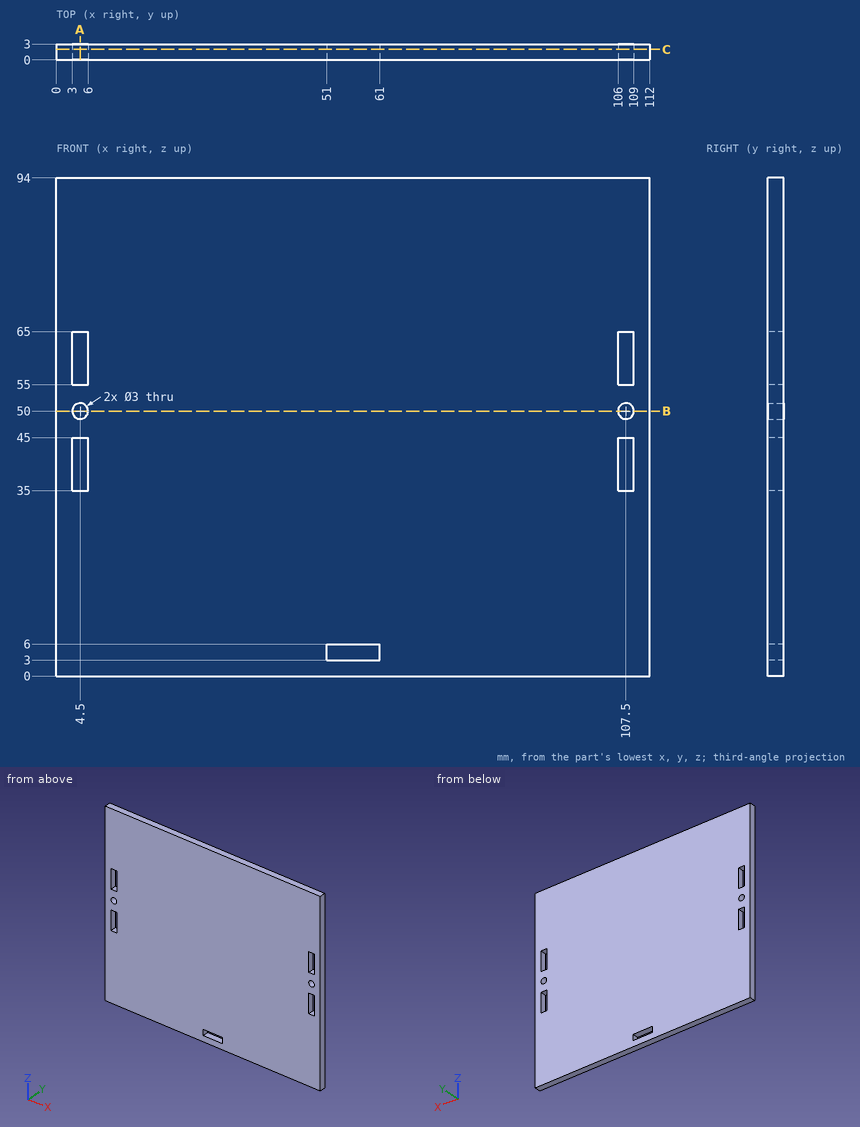
Geometry check sheet. Reference: drawing and pictorial views, mm from the part's lowest x, y, z. Round coordinates to 2 decimals unless told otherwise and drop trailing zeros. Loops run counter-clockwise (first coordinate to the right, second up) from the corner with the lowest first, then second, coordinate; pieces in that order, holes last. Notation, with made-up numbers: (-10.5, 12.25) -> (23.5, 12.25) arc R18 cw to (23.5, 25.25) -> close; hole circle Ø11 at (25, 54.5). An arc over 180 degrees is marked (long way). Answer as a JSON object with one key per item and string values. Group by question number.
Item 1: Depth check by flat-ended pin: pin 1 Ø1.8 at (x, z) = (107.5, 50) entering from +Y. Enter the tip coordinate at first touch or a pass-through.
Item 2: Cross-section at B-B, the plane z = 50. Record the cut outline in (x, y).
Item 3: Cross-section at C-C, the plane y = 2. Record the cut outline in (x, z).
Item 4: Cross-section at A-A, the plane x = 4.5. Record the cut outline in (y, z), plus the area to 3 significant figures.
Item 5: Thickness scan on line 1 along X through (y, z) = (2.2, 60.5); line 2 along Z through (x, y) = (4.5, 2.3); line 3 along Z through (x, y) = (55.5, 2.35). Record the ranges inside material, lowest first.
Determined:
{
 "1": {"pin 1": "passes through"},
 "2": {"outline": "(0, 0) -> (3, 0) -> (3, 3) -> (0, 3) -> close; (6, 0) -> (106, 0) -> (106, 3) -> (6, 3) -> close; (109, 0) -> (112, 0) -> (112, 3) -> (109, 3) -> close"},
 "3": {"outline": "(0, 0) -> (112, 0) -> (112, 94) -> (0, 94) -> close; hole (3, 35) -> (6, 35) -> (6, 45) -> (3, 45) -> close; hole circle Ø3 at (4.5, 50); hole (3, 55) -> (6, 55) -> (6, 65) -> (3, 65) -> close; hole (51, 3) -> (61, 3) -> (61, 6) -> (51, 6) -> close; hole (106, 35) -> (109, 35) -> (109, 45) -> (106, 45) -> close; hole circle Ø3 at (107.5, 50); hole (106, 55) -> (109, 55) -> (109, 65) -> (106, 65) -> close"},
 "4": {"outline": "(0, 0) -> (3, 0) -> (3, 35) -> (0, 35) -> close; (0, 45) -> (3, 45) -> (3, 48.5) -> (0, 48.5) -> close; (0, 51.5) -> (3, 51.5) -> (3, 55) -> (0, 55) -> close; (0, 65) -> (3, 65) -> (3, 94) -> (0, 94) -> close", "area": "213 mm²"},
 "5": {"line 1": "x = 0 to 3, 6 to 106, 109 to 112", "line 2": "z = 0 to 35, 45 to 48.5, 51.5 to 55, 65 to 94", "line 3": "z = 0 to 3, 6 to 94"}
}
